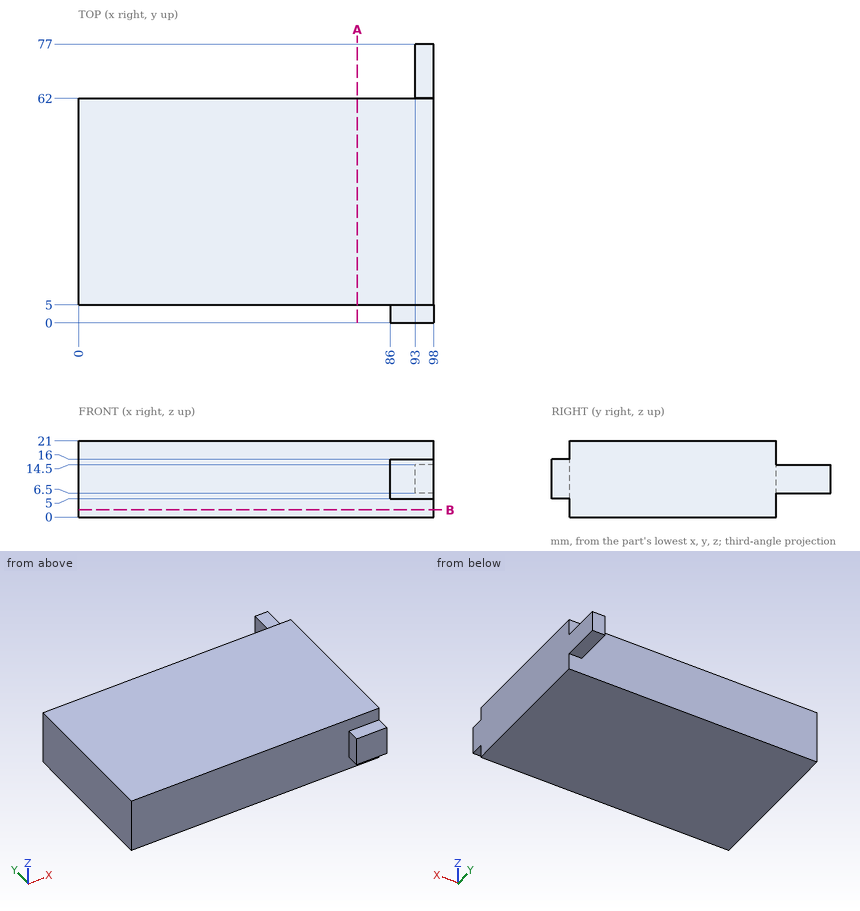
Design review of the part shown in the three views and the two pictorial views. Dimensions are in mm from the part's minimum x, y and z. Round coordinates to 2 decimals unless told otherwise and drop trailing zeros. Loops run counter-clockwise (first coordinate to the right, second up) from the corner with the lowest first, then second, coordinate; pieces in that order, holes last. Notation, with made-up numbers: (25, 30) -> (51, 30) arc R24 ccw to (51, 58) -> close; hole circle Ø5 at (77.5, 84.25). An arc over 180 degrees is marked (long way). Return JSON: item names as keys, results as strings.
(1) For pin 1 (10 mm diameter, centred on x = 74, z = 2.5, fed in from -Y); pin 2 (6.5 mm diameter, centred on x = 27.5, z = 7.5, fed in from +Y); pin 3 (4 mm diameter, centred on x = 94, y = 1.5, fed in from -Z), all flat-tipped, find the tip position at first contact; note any pin that passes through.
Solved:
{"pin 1": "y = 5", "pin 2": "y = 62", "pin 3": "z = 5"}
(2) For line 1 (Y direction, x = 65, z = 10.5), list the stretches that pass through material, from the lowest coordinate up.
Solved:
{"line 1": "5 to 62"}
(3) Add section A-A on x = 77. Write out the cut boundary in (y, z), plus the area to 3 significant figures.
Solved:
{"outline": "(5, 0) -> (62, 0) -> (62, 21) -> (5, 21) -> close", "area": "1,200 mm2"}
(4) Add section B-B on z = 2. Write out the cut boundary in (x, y), plus the area to 3 significant figures.
Solved:
{"outline": "(0, 5) -> (98, 5) -> (98, 62) -> (0, 62) -> close", "area": "5,590 mm2"}
